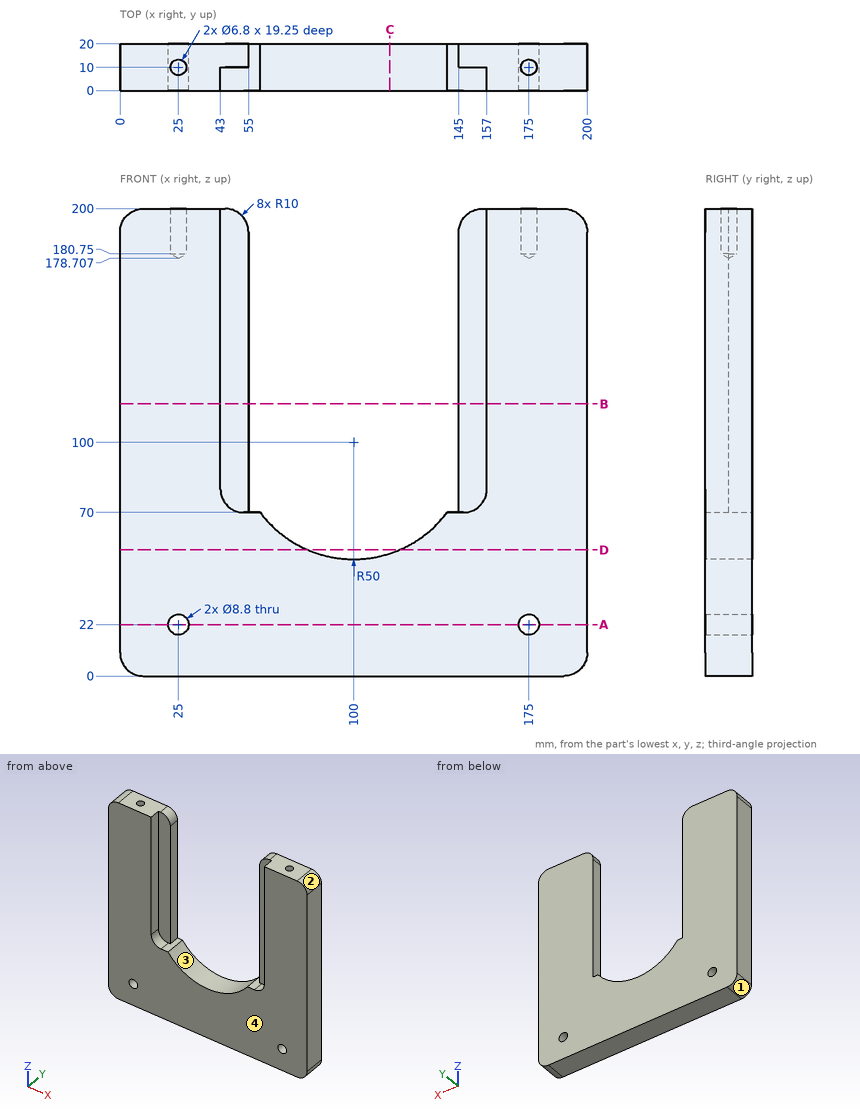
Can you work these out from the drawing? Everything is in mm from the part's minimum corner. Give positions to 0.01 mm unless a question says otherwise; leave off trailing zeros. Order: outer loops, then holes, each group sorted by start corner. A loop starts at its lowest first (then second) coordinate and runs counter-clockwise, first axis right, second up. Notation, with made-up numbers: M 37.5,69 L 60.5,69 A12 ccw 60.5,86 Z; hole C 13.5,-35 d3. An arc over 180 degrees is marked long. One line per item, written item: value.
Item 1: If we section it at A-A on z = 22: Write out the boundary of the cut face in (x, y), and give its area (3 significant figures).
Verdict:
outline: M 0,0 L 20.6,0 L 20.6,20 L 0,20 Z; M 29.4,0 L 170.6,0 L 170.6,20 L 29.4,20 Z; M 179.4,0 L 200,0 L 200,20 L 179.4,20 Z
area: 3,650 mm2
Item 2: If we section it at D-D on z = 54: Write out the boundary of the cut face in (x, y), and give its area (3 significant figures).
Verdict:
outline: M 0,0 L 80.4,0 L 80.4,20 L 0,20 Z; M 119.6,0 L 200,0 L 200,20 L 119.6,20 Z
area: 3,220 mm2
Item 3: If we section it at C-C on x = 115.5: Write out the boundary of the cut face in (y, z).
Verdict:
outline: M 0,0 L 20,0 L 20,52.46 L 0,52.46 Z
Item 4: For pin 1 (6 mm diameter, centred on x = 48.5, y = 2.5, fed in from +Z); pin 2 (3.5 mm diameter, centred on x = 55.5, y = 8, fed in from +Z); pin 3 (3.5 mm diameter, centred on x = 152, z = 160, fed in from -Y), each with a flat end and sliding along its axis, tell me the tip position at first contact or that it passes through.
Verdict:
pin 1: z = 73.39
pin 2: z = 70
pin 3: y = 10
Item 5: If we section it at B-B on z = 116.5: Write out the boundary of the cut face in (x, y), and give its area (3 significant figures).
Verdict:
outline: M 0,0 L 43,0 L 43,10 L 55,10 L 55,20 L 0,20 Z; M 145,10 L 157,10 L 157,0 L 200,0 L 200,20 L 145,20 Z
area: 1,960 mm2
Item 6: If we mould it in two halves opening along X, with no side actions, what happens to the marked faces 1, 2, 3 and 4? For each: pulls with the +X half, pulls with the -X half, needs draft (parallel to the pull), parting line crosses it, or undercut.
Verdict:
face 1: pulls with the -X half
face 2: pulls with the +X half
face 3: undercut
face 4: needs draft
Item 7: Please list where these lines run through material, in increasing order: line 1 (X direction, y = 2, z = 164); line 2 (X direction, y = 16, z = 87); line 3 (Y direction, x = 25, z = 186).
Verdict:
line 1: 0 to 43, 157 to 200
line 2: 0 to 55, 145 to 200
line 3: 0 to 6.6, 13.4 to 20
